Input: part model. Units: mm. Frame: model coordinates. Face numbers are marked on the shaded views. A direction names the side the tool comes from. Give positions to 0.01 mm unless a question says otherwise; leave off trailing zeros. Loops run counter-clockwise (first coordinate to the right, second up) from the corner with the lowest first, then second, coordinate; pieces in that order, holes last. Notation, with made-up numbers: (50, -32.5) - (64, -32.5) arc R14 cw to (64, -26.5) - close; hole circle Ø7 at (27, -19.5). An arc over 180 degrees is marked (long way). Answer as a JSON object with one key per item and string values. Group by question number.
(1) Section query A-A (x = 0). Return loops of the section in (y, z).
(2) Material intervals for L1, parallel to X at y = 2, z = 18; L2, parallel to Z at x = -13.5, y = 2.55; L3, parallel to X at y = 1.5, z = 5, sorted ascending.
(3) Access query for the marked faces 1 and 2. Directions: +Z, -Z, +X, -X, +Y, -Y. A direction counts if a zero-diameter tool reaches every point of the face in a straight line with its end or side. Return the directions, or none.
(4) Section query C-C (y = 0.75). Count the separate pieces of the cut face and the enclosed holes in it, plus the area to 3 significant figures.
(5) Mould query, pull axis Z, two halves, no side actions, for the marked faces 3, 4, 5 and 6. Classes: +Z half, -Z half, draft (parallel to the pull), parting line (faces both ways), or undercut.
(6) Pin query (flat end, axial travel): P1, Ø1.5, axis at x = 13, y = 0.5, coming from the +Z side; P2, Ø3, axis at x = 12.7, z = 19.05, coming from the +Y side. Return the tip coordinate at first contact, or that it passes through.
(7) Section query B-B (z = 19.05). Return loops of the section in (x, y).
(8) Section query D-D (x = -11.5). Return loops of the section in (y, z).
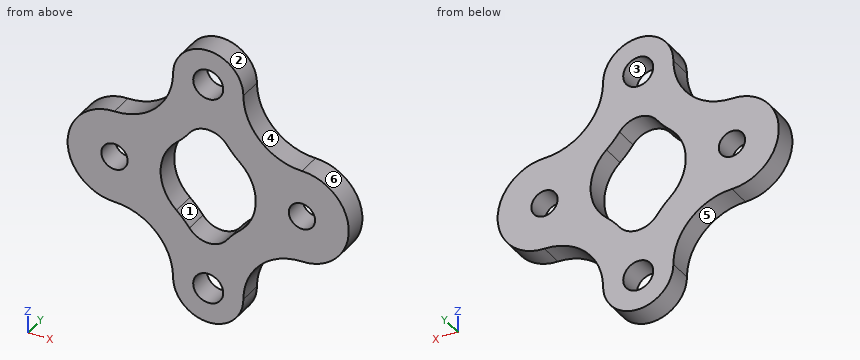
```python
from build123d import *

# Parameters (mm, degrees)
BOSS_EXTRUDE1_DEPTH = 3.175254
SKETCH2_R           = 2.032
SKETCH2_R_2         = 1.778
CUT_EXTRUDE1_DEPTH  = 43.71527523
CUT_EXTRUDE2_DEPTH  = 43.71527523


with BuildPart() as part:
    # Sketch1 → Boss-Extrude1 (new body)
    with BuildSketch(Plane(origin=(0, 0, 0), x_dir=(1, 0, 0), z_dir=(0, 1, 0))):
        with BuildLine():
            ThreePointArc((4.7625, -4.7625), (0, 0), (-4.7625, -4.7625))
            ThreePointArc((-4.7625, -4.7625), (-7.087339924, -10.375160076), (-12.7, -12.7))
            ThreePointArc((-12.7, -12.7), (-19.05, -19.05), (-12.7, -25.4))
            ThreePointArc((-12.7, -25.4), (-7.087339924, -27.724839924), (-4.7625, -33.3375))
            ThreePointArc((-4.7625, -33.3375), (0, -38.1), (4.7625, -33.3375))
            ThreePointArc((4.7625, -33.3375), (7.087339924, -27.724839924), (12.7, -25.4))
            ThreePointArc((12.7, -25.4), (19.05, -19.05), (12.7, -12.7))
            ThreePointArc((12.7, -12.7), (7.087339924, -10.375160076), (4.7625, -4.7625))
        make_face()
    extrude(amount=BOSS_EXTRUDE1_DEPTH)

    # Sketch2 → Cut-Extrude1 (cut, through all)
    with BuildSketch(Plane(origin=(0, 3.175254, 0), x_dir=(1, 0, 0), z_dir=(0, 1, 0))):
        with Locations(Location((0, -4.7625, 0), (0, 0, 270))):
            Circle(SKETCH2_R)
        with Locations(Location((12.7, -19.05, 0), (0, 0, 270))):
            Circle(SKETCH2_R_2)
        with Locations(Location((0, -33.3375, 0), (0, 0, 270))):
            Circle(SKETCH2_R)
        with Locations(Location((-12.7, -19.05, 0), (0, 0, 270))):
            Circle(SKETCH2_R_2)
    extrude(amount=-CUT_EXTRUDE1_DEPTH, mode=Mode.SUBTRACT)

    # Sketch3 → Cut-Extrude2 (cut, through all)
    with BuildSketch(Plane(origin=(0, 3.175254, 0), x_dir=(1, 0, 0), z_dir=(0, 1, 0))):
        with BuildLine():
            ThreePointArc((-4.299739587, -14.2875), (-6.449609381, -19.05), (-4.299739587, -23.8125))
            ThreePointArc((-4.299739587, -23.8125), (-3.371116203, -24.719963977), (-2.54, -25.7175))
            ThreePointArc((-2.54, -25.7175), (0, -26.9875), (2.54, -25.7175))
            ThreePointArc((2.54, -25.7175), (3.371116203, -24.719963977), (4.299739587, -23.8125))
            ThreePointArc((4.299739587, -23.8125), (6.449609381, -19.05), (4.299739587, -14.2875))
            ThreePointArc((4.299739587, -14.2875), (3.371116203, -13.380036023), (2.54, -12.3825))
            ThreePointArc((2.54, -12.3825), (0, -11.1125), (-2.54, -12.3825))
            ThreePointArc((-2.54, -12.3825), (-3.371116203, -13.380036023), (-4.299739587, -14.2875))
        make_face()
    extrude(amount=-CUT_EXTRUDE2_DEPTH, mode=Mode.SUBTRACT)


solid = part.part
```
Recorded:
{
 "1": {"outline": "(0, 0) - (3.18, 0) - (3.18, 2.73) - (0, 2.73) - close; (0, 6.79) - (3.18, 6.79) - (3.18, 11.11) - (0, 11.11) - close; (0, 26.99) - (3.18, 26.99) - (3.18, 31.31) - (0, 31.31) - close; (0, 35.37) - (3.18, 35.37) - (3.18, 38.1) - (0, 38.1) - close"},
 "2": {"L1": "x = -18.96 to -14.13, -11.27 to -6.36, 6.36 to 11.27, 14.13 to 18.96", "L2": "z = 12.75 to 17.46, 20.64 to 25.35", "L3": "x = -4.77 to -2.02, 2.02 to 4.77"},
 "3": {"face 1": "+Y, -Y", "face 2": "+Z, +Y, -Y"},
 "4": {"separate pieces": "1", "enclosed holes": "5", "area": "535 mm^2"},
 "5": {"face 3": "undercut", "face 4": "+Z half", "face 5": "-Z half", "face 6": "parting line"},
 "6": {"P1": "stops at z = 25.41", "P2": "passes through"},
 "7": {"outline": "(-19.05, 0) - (-14.48, 0) - (-14.48, 3.18) - (-19.05, 3.18) - close; (-10.92, 0) - (-6.45, 0) - (-6.45, 3.18) - (-10.92, 3.18) - close; (6.45, 0) - (10.92, 0) - (10.92, 3.18) - (6.45, 3.18) - close; (14.48, 0) - (19.05, 0) - (19.05, 3.18) - (14.48, 3.18) - close"},
 "8": {"outline": "(0, 12.61) - (3.18, 12.61) - (3.18, 17.74) - (0, 17.74) - close; (0, 20.36) - (3.18, 20.36) - (3.18, 25.49) - (0, 25.49) - close"}
}
